```python
from build123d import *

# Parameters (mm, degrees)
F0_W     = 60
F0_H     = 28
F1_DEPTH = 40
F2_W     = 42
F2_H     = 28
F3_DEPTH = 12
F4_R     = 10
F5_DEPTH = 60
F6_W     = 12
F6_H     = 28
F7_DEPTH = 30


with BuildPart() as f1:
    # F0 (on Top) → F1 (new body)
    with BuildSketch(Plane.XY):
        with Locations((-28.556031, -25.896984)):
            Rectangle(F0_W, F0_H)
    extrude(amount=F1_DEPTH)

    # F2 (on face) → F3 (cut)
    with BuildSketch(Plane.XY.offset(40)):
        with Locations((-19.556031, -25.896984)):
            Rectangle(F2_W, F2_H)
    extrude(amount=-F3_DEPTH, mode=Mode.SUBTRACT)

    # F4 (on face) → F5 (cut)
    with BuildSketch(Plane.YZ.offset(1.443969)):
        with Locations((-25.896984, 14)):
            Circle(F4_R)
    extrude(amount=-F5_DEPTH, mode=Mode.SUBTRACT)

    # F6 (on face) → F7 (cut)
    with BuildSketch(Plane.YZ.offset(1.443969)):
        with Locations((-25.896984, 14)):
            Rectangle(F6_W, F6_H)
    extrude(amount=-F7_DEPTH, mode=Mode.SUBTRACT)


solid = f1.part
```
Geometry: final body of the model. Coordinates: model frame, mm. A direction names the side the tool comes from. Round coordinates to 2 decimals unless told otherwise and drop trailing zeros. Write each loop counter-clockwise with the first axis right and the second up, starting at its lowest first coordinate (ties: lowest second). Pieces come first, ordered by that corner, then holes. Notation, with made-up numbers: M 66.5,80.5 L 124.5,80.5 A5 ccw 124.5,87.5 Z; hole C 39,5.25 d2. An arc over 180 degrees is marked long. Answer in a Markdown table with one row per item. Add a question column.
(1) Reachability of faces 1 (the face through (-28.556, -26, 26)), 2 (the face through (-34.803, -35.887, 14.44)), 3 (the face through (-20, -19, 28)) from +Z, -Z, +X, -X, +Y, -Y: full face, straight path, thin tool, end or side. Return the list, or none.
(2) Cut plane C-C, the plane z = 14. Return the cut outline in (x, y), then the cut area to 3 significant figures.
(3) Contact query for flat-ended pins moving along their axis: pin 1 (8 mm diameter, centred on y = -27, z = 18, fed in from -X); pin 2 (14 mm diameter, centred on x = -24, y = -25, fed in from +Z); pin 3 (3 mm diameter, centred on y = -24, z = 2, fed in from +X); pin 4 (9.5 mm diameter, centred on y = -27, z = 33.5, fed in from +X). Output: stop coordinate, or through.
(4) Ray query, L1, parallel to Y at x = -3.5, z = 26.5; L2, parallel to Z at x = -36.5, y = -25.75; L3, parallel to X at y = -26, z = 36.5. Return the intervals inside material, ascending.
(5) Cut plane B-B, the plane y = -18.75. Return the cut outline in (x, z), then the cut area to 3 significant figures.
(6) Cut plane D-D, the plane y = -14.75. Return the cut outline in (x, z), then the cut area to 3 significant figures.
(7) Cut plane A-A, the plane x = -24. Return the cut outline in (y, z), then the cut area to 3 significant figures.
(8) Draft query along Y for faces 4 (the face through (-29, -11.897, 15)), 5 (the face through (-13, -19.897, 25)), 6 (the face through (1.444, -15, 14)). Return one class per face: pulls with the +Y half, pulls with the -Y half, needs draft (parallel to the pull), parting line crosses it, or undercut.
Established:
| question | item | result |
|---|---|---|
| 1 | face 1 | +Z, -Z, +X |
| 1 | face 2 | +X, -X |
| 1 | face 3 | +Z, +X, +Y, -Y |
| 2 | outline | M -58.56,-39.9 L 1.44,-39.9 L 1.44,-35.9 L -58.56,-35.9 Z; M -58.56,-15.9 L 1.44,-15.9 L 1.44,-11.9 L -58.56,-11.9 Z |
| 2 | area | 480 mm² |
| 3 | pin 1 | through |
| 3 | pin 2 | z = 28 |
| 3 | pin 3 | x = -28.56 |
| 3 | pin 4 | x = -40.56 |
| 4 | L1 | -39.9 to -31.9, -19.9 to -11.9 |
| 4 | L2 | 0 to 4, 24 to 28 |
| 4 | L3 | -58.56 to -40.56 |
| 5 | outline | M -58.56,0 L 1.44,0 L 1.44,7.01 L -58.56,7.01 Z; M -58.56,20.99 L 1.44,20.99 L 1.44,28 L -40.56,28 L -40.56,40 L -58.56,40 Z |
| 5 | area | 1,060 mm² |
| 6 | outline | M -58.56,0 L 1.44,0 L 1.44,28 L -40.56,28 L -40.56,40 L -58.56,40 Z |
| 6 | area | 1,900 mm² |
| 7 | outline | M -39.9,0 L -31.9,0 L -31.9,6 A10 cw -31.9,22 L -31.9,28 L -39.9,28 Z; M -19.9,0 L -11.9,0 L -11.9,28 L -19.9,28 L -19.9,22 A10 cw -19.9,6 Z |
| 7 | area | 359 mm² |
| 8 | face 4 | pulls with the +Y half |
| 8 | face 5 | undercut |
| 8 | face 6 | needs draft |
